```python
from build123d import *

# Parameters (mm, degrees)
F0_W     = 40
F0_H     = 50
F1_DEPTH = 50
F2_R     = 20
F3_SIZE  = 5
F4_T     = -2.5
F6_R     = 12.5
F7_DEPTH = 2.5


with BuildPart() as f1:
    # F0 (on Front) → F1 (new body)
    with BuildSketch(Plane.XZ):
        with Locations((9.33321, 13.938332)):
            Rectangle(F0_W, F0_H)
    extrude(amount=F1_DEPTH)

    # F2
    f2_edges = [f1.edges().sort_by_distance(p)[0] for p in [
        (9.33321, -50, 38.938332),
        (29.33321, -25, -11.061668),
    ]]
    fillet(f2_edges, radius=F2_R)

    # F3
    f3_edges = [f1.edges().sort_by_distance(p)[0] for p in [
        (29.33321, -15, 38.938332),
    ]]
    chamfer(f3_edges, length=F3_SIZE)

    # F4
    f4_openings = [f1.faces().sort_by_distance(p)[0] for p in [
        (8.511559, 0, 14.711798),
    ]]
    offset(amount=F4_T, openings=f4_openings)

    # F5: F1 across plane


with BuildPart() as f1_1:
    add(f1.part)
    add(f1.part.mirror(Plane.XZ))

    # F6 (on face) → F7 (cut, through all)
    with BuildSketch(Plane(origin=(-10.66679, 0, 0), x_dir=(0, -1, 0), z_dir=(-1, 0, 0))):
        with Locations((0, 12.662414)):
            Circle(F6_R)
    extrude(amount=-F7_DEPTH, mode=Mode.SUBTRACT)


solid = f1_1.part
```
The listing builds one solid part. Answer for the finished solid, in the listing's coordinates (mm). A direction names the side the tool comes from. Coordinates: 2 decimals unless noted, no trailing zeros. Write each loop counter-clockwise with the first axis right and the second up, starting at its lowest first coordinate (ties: lowest second). Pieces come first, ordered by that corner, then holes.
Q1. Given P1, Ø10, axis at y = 6, z = 10, coming from the -X side; P2, Ø8, axis at x = 22.5, z = 30.5, coming from the +Y side; P3, Ø4, axis at y = 4.5, z = 3.5, coming from the -X side, each flat-ended and moving along its own axis, determine where each tip first touches the part or whether it passes through.
Returned:
P1: stops at x = 26.38
P2: stops at y = 48.52
P3: stops at x = 25.17
Q2. The mould has two halves that part along X. Classify faces 4 (the cylindrical face through (7.786, -42.238, 31.448)), 5 (the conical face through (27.979, -41.436, 30.629)), 6 (the cylindrical face through (7.078, -43.986, 33.235)): released by +X, released by -X, zero draft, split by the parting line, or undercut.
Returned:
face 4: undercut
face 5: released by +X
face 6: zero draft
Q3. Which of the six approach directions +Z, -Z, +X, -X, +Y, -Y give full straight-line access (tool end or side, diameter ignored) to faces 1 (the flat face through (26.833, -1, 21)), 2 (the flat face through (-1, -1, -11.062)), 3 (the cylindrical face through (-9.43, 2.71, 0.46))?
Returned:
face 1: none
face 2: -Z, +X, -X, +Y, -Y
face 3: -X
Q4. Section B-B, the plane y = 27 is taken. Write down the section's boundary in (x, z), then the cut area to 3 significant figures.
Returned:
outline: (-10.67, -11.06) - (9.33, -11.06) arc R20 ccw to (29.33, 8.94) - (29.33, 33.94) - (24.33, 38.94) - (-10.67, 38.94) - close; hole (-8.17, -8.56) - (9.33, -8.56) arc R17.5 ccw to (26.83, 8.94) - (26.83, 32.9) - (23.3, 36.44) - (-8.17, 36.44) - close
area: 399 mm2
Q5. Section C-C, the plane z = 15 is taken. Write down the section's boundary in (x, y).
Returned:
outline: (-10.67, -50) - (24.33, -50) - (29.33, -45) - (29.33, 45) - (24.33, 50) - (-10.67, 50) - (-10.67, 12.28) - (-8.17, 12.28) - (-8.17, 47.5) - (23.3, 47.5) - (26.83, 43.96) - (26.83, -43.96) - (23.3, -47.5) - (-8.17, -47.5) - (-8.17, -12.28) - (-10.67, -12.28) - close
Q6. Section D-D, the plane y = 0 is taken. Write down the section's boundary in (x, z).
Returned:
outline: (-10.67, -11.06) - (9.33, -11.06) arc R20 ccw to (29.33, 8.94) - (29.33, 33.94) - (24.33, 38.94) - (-10.67, 38.94) - (-10.67, 25.16) - (-8.17, 25.16) - (-8.17, 36.44) - (23.3, 36.44) - (26.83, 32.9) - (26.83, 8.94) arc R17.5 cw to (9.33, -8.56) - (-8.17, -8.56) - (-8.17, 0.16) - (-10.67, 0.16) - close
Q7. Section A-A, the plane x = -3.5 is taken. Write down the section's boundary in (y, z), then the cut area to 3 significant figures.
Returned:
outline: (-50, -6.06) - (-45, -11.06) - (45, -11.06) - (50, -6.06) - (50, 18.94) arc R20 ccw to (30, 38.94) - (-30, 38.94) arc R20 ccw to (-50, 18.94) - close; hole (-47.5, -5.03) - (-43.96, -8.56) - (43.96, -8.56) - (47.5, -5.03) - (47.5, 18.94) arc R17.5 ccw to (30, 36.44) - (-30, 36.44) arc R17.5 ccw to (-47.5, 18.94) - close
area: 672 mm2
Q8. Find the intervals of material crossed by line 1 along Z through (x, y) = (-8.75, 0); line 2 along Y through (x, z) = (-3.5, 19); line 3 along X through (y, z) = (15, 31), in increasing order.
Returned:
line 1: z = -11.06 to 0.16, 25.16 to 38.94
line 2: y = -50 to -47.5, 47.5 to 50
line 3: x = -10.67 to -8.17, 26.83 to 29.33
